from build123d import *

# Parameters (mm, degrees)
BOSS_EXTRUDE1_DEPTH = 106
BOSS_EXTRUDE2_DEPTH = 3
SKETCH3_R           = 2.5
BOSS_EXTRUDE3_DEPTH = 3.5
CUT_EXTRUDE1_DEPTH  = 16.5
FILLET1_R           = 5


with BuildPart() as part:
    # Sketch1 → Boss-Extrude1 (new body)
    with BuildSketch(Plane(origin=(0, 0, 0), x_dir=(1, 0, 0), z_dir=(0, 1, 0))):
        with BuildLine():
            Line((83, -33), (-83, -33))
            ThreePointArc((-83, -33), (-86.535533906, -31.535533906), (-88, -28))
            Line((-88, -28), (-88, 28))
            ThreePointArc((-88, 28), (-86.535533906, 31.535533906), (-83, 33))
            Line((-83, 33), (83, 33))
            ThreePointArc((83, 33), (86.535533906, 31.535533906), (88, 28))
            Line((88, 28), (88, -28))
            ThreePointArc((88, -28), (86.535533906, -31.535533906), (83, -33))
        make_face()
        with BuildLine():
            Line((80, -30), (-80, -30))
            ThreePointArc((-80, -30), (-83.535533906, -28.535533906), (-85, -25))
            Line((-85, -25), (-85, 25))
            ThreePointArc((-85, 25), (-83.535533906, 28.535533906), (-80, 30))
            Line((-80, 30), (80, 30))
            ThreePointArc((80, 30), (83.535533906, 28.535533906), (85, 25))
            Line((85, 25), (85, -25))
            ThreePointArc((85, -25), (83.535533906, -28.535533906), (80, -30))
        make_face(mode=Mode.SUBTRACT)
    extrude(amount=BOSS_EXTRUDE1_DEPTH)

    # Sketch2 → Boss-Extrude2 (add)
    with BuildSketch(Plane(origin=(0, 106, 0), x_dir=(1, 0, 0), z_dir=(0, 1, 0))):
        with BuildLine():
            Line((-83, 33), (83, 33))
            ThreePointArc((83, 33), (86.535533906, 31.535533906), (88, 28))
            Line((88, 28), (88, -28))
            ThreePointArc((88, -28), (86.535533906, -31.535533906), (83, -33))
            Line((83, -33), (-83, -33))
            ThreePointArc((-83, -33), (-86.535533906, -31.535533906), (-88, -28))
            Line((-88, -28), (-88, 28))
            ThreePointArc((-88, 28), (-86.535533906, 31.535533906), (-83, 33))
        make_face()
    extrude(amount=BOSS_EXTRUDE2_DEPTH)

    # Sketch3 → Boss-Extrude3 (add)
    with BuildSketch(Plane.XZ):
        with BuildLine():
            Line((-83, 33), (83, 33))
            Line((83, 33), (83, 38))
            ThreePointArc((83, 38), (81.535533906, 41.535533906), (78, 43))
            Line((78, 43), (-78, 43))
            ThreePointArc((-78, 43), (-81.535533906, 41.535533906), (-83, 38))
            Line((-83, 38), (-83, 33))
        make_face()
        with Locations(Location((-60, 38, 0), (0, 0, 270))):
            Circle(SKETCH3_R, mode=Mode.SUBTRACT)
        with Locations(Location((60, 38, 0), (0, 0, 90))):
            Circle(SKETCH3_R, mode=Mode.SUBTRACT)
    boss_extrude3 = extrude(amount=-BOSS_EXTRUDE3_DEPTH)

    # Mirror1: Boss-Extrude3 across plane
    add(boss_extrude3.mirror(Plane.XY))

    # Sketch4 → Cut-Extrude1 (cut, symmetric)
    with BuildSketch(Plane(origin=(0, 0, -33), x_dir=(-1, 0, 0), z_dir=(0, 0, -1))):
        with BuildLine():
            Line((47.5, -56), (-47.5, -56))
            Line((-47.5, -56), (-47.5, 51))
            ThreePointArc((-47.5, 51), (-46.035533906, 54.535533906), (-42.5, 56))
            Line((-42.5, 56), (42.5, 56))
            ThreePointArc((42.5, 56), (46.035533906, 54.535533906), (47.5, 51))
            Line((47.5, 51), (47.5, -56))
        make_face()
    extrude(amount=CUT_EXTRUDE1_DEPTH, both=True, mode=Mode.SUBTRACT)

    # Fillet1
    fillet1_edges = [part.edges().sort_by_distance(p)[0] for p in [
        (47.5, 1.75, -43),
        (-47.5, 1.75, -43),
    ]]
    fillet(fillet1_edges, radius=FILLET1_R)


solid = part.part
The model under review builds one solid part; all positions refer to its coordinate system, in mm. A direction names the side the tool comes from. Coordinates: 2 decimals unless noted, no trailing zeros. Loops run counter-clockwise (first coordinate to the right, second up) from the corner with the lowest first, then second, coordinate; pieces in that order, holes last. Notation, with made-up numbers: M -19.75,44 L 4.25,44 A19 ccw 4.25,74 Z; hole C -20,52 d7. An arc over 180 degrees is marked long. Put each result on its own line as item: value. Start each with the question number.
Q1. Add section D-D (y = 48.5). Write out the cut boundary in (x, z).
Q2. Add section C-C (z = -23). Write out the cut boundary in (x, y).
Q3. Add section A-A (x = 60). Write out the cut boundary in (y, z).
Q4. The part is to be moulded in two halves that separate along X. For faces 1 (the cylindrical face through (83, 52, -29)), 2 (the cylindrical face through (86, 54, -32)), 3 (the flat face through (-7, 0, 32)), say which applies: +X half, -X half, draft (parallel to the pull), parting line (faces both ways), or undercut.
Q5. For faces 4 (the cylindrical face through (48.93, 1.73, -41.5)), 5 (the flat face through (-65, 3.5, -38)), 6 (the flat face through (83, 2, -35)), 7 (the cylindrical face through (-84, 52, -28)), list the 3-axis set-ups (+Z, -Z, +X, -X, +Y, -Y) from which the entire face can be reached by the end or side of a thin tool; tool diameter is ignored.
Q6. Wall thickness on line 1 (Z direction, x = 60, y = 1.2); line 2 (X direction, y = 2.1, z = -38); line 3 (X direction, y = 2.5, z = 38): over which ranges is each line inside the solid? List them lowest first.
Q7. Add section B-B (y = 92). Write out the cut boundary in (x, z), and give its area (3 significant figures).
Q8. Clearance check with flat-ended pins moving along their axes: pin 1 (12 mm diameter, centred on x = 30, z = 17.5, fed in from -Y); pin 2 (6.5 mm diameter, centred on y = 24, z = -35.5, fed in from +X); pin 3 (3 mm diameter, centred on x = 56, y = 32, fed in from -Z); pin 4 (4 mm diameter, centred on x = -60, z = -38, fed in from -Y). State where each tip first meets the part, or that it passes through.
Answers:
1. outline: M -88,-28 A5 ccw -83,-33 L -47.5,-33 L -47.5,-30 L -80,-30 A5 cw -85,-25 L -85,25 A5 cw -80,30 L 80,30 A5 cw 85,25 L 85,-25 A5 cw 80,-30 L 47.5,-30 L 47.5,-33 L 83,-33 A5 ccw 88,-28 L 88,28 A5 ccw 83,33 L -83,33 A5 ccw -88,28 Z
2. outline: M -88,0 L -85,0 L -85,106 L 85,106 L 85,0 L 88,0 L 88,109 L -88,109 Z
3. outline: M 0,-43 L 3.5,-43 L 3.5,-40.5 L 0,-40.5 Z; M 0,-35.5 L 3.5,-35.5 L 3.5,-33 L 109,-33 L 109,33 L 3.5,33 L 3.5,35.5 L 0,35.5 L 0,30 L 106,30 L 106,-30 L 0,-30 Z; M 0,40.5 L 3.5,40.5 L 3.5,43 L 0,43 Z
4. face 1: undercut
4. face 2: +X half
4. face 3: draft
5. face 4: -Z, +Y, -Y
5. face 5: -Z, +X, -X, +Y
5. face 6: -Z, +X, +Y, -Y
5. face 7: -Y
6. line 1: z = -43 to -40.5, -35.5 to -30, 30 to 35.5, 40.5 to 43
6. line 2: x = -83 to -62.5, -57.5 to -47.5, 47.5 to 57.5, 62.5 to 83
6. line 3: x = -83 to -62.5, -57.5 to 57.5, 62.5 to 83
7. outline: M -88,-28 A5 ccw -83,-33 L 83,-33 A5 ccw 88,-28 L 88,28 A5 ccw 83,33 L -83,33 A5 ccw -88,28 Z; hole M -85,-25 A5 ccw -80,-30 L 80,-30 A5 ccw 85,-25 L 85,25 A5 ccw 80,30 L -80,30 A5 ccw -85,25 Z
7. area: 1,420 mm^2
8. pin 1: stops at y = 106
8. pin 2: stops at x = 85.63
8. pin 3: stops at z = -33
8. pin 4: passes through
